from build123d import *

# Parameters (mm, degrees)
PAD_DEPTH       = 129
FILLET_R        = 3
FILLET001_R     = 2
POCKET_DEPTH    = 29.348127
SKETCH002_W     = 23
SKETCH002_H     = 7
POCKET001_DEPTH = 49


with BuildPart() as obj1:
    # Sketch → Pad (new body)
    with BuildSketch(Plane.XZ):
        with BuildLine():
            Line((0, 0), (0, 37))
            Line((0, 37), (3, 44))
            Line((3, 44), (3, 4))
            Line((3, 4), (26, 4))
            Line((26, 4), (21, 34))
            ThreePointArc((23.448856, 44), (21.197055, 39.251589), (21, 34))
            ThreePointArc((25.84203, 42.190943), (25.551614, 44.294231), (23.448856, 44))
            ThreePointArc((25.84203, 42.190943), (24.041555, 38.293355), (24.041381, 34))
            Line((24.041381, 34), (29.708048, 0))
            Line((29.708048, 0), (0, 0))
        make_face()
    extrude(amount=PAD_DEPTH)

    # Fillet
    fillet_edges = [obj1.edges().sort_by_distance(p)[0] for p in [
        (26, -64.5, 4),
        (3, -64.5, 4),
    ]]
    fillet(fillet_edges, radius=FILLET_R)

    # Fillet001
    fillet001_edges = [obj1.edges().sort_by_distance(p)[0] for p in [
        (0, -64.5, 0),
        (29.708048, -64.5, 0),
    ]]
    fillet(fillet001_edges, radius=FILLET001_R)

    # Sketch001 (on Face2 of Fillet001) → Pocket (cut, through all)
    with BuildSketch(Plane(origin=(0, 0, 0), x_dir=(0, 0, -1), z_dir=(-1, 0, 0))):
        Polygon((0, 49), (-45, 4), (-45, 0), (0, 0), align=None)
    extrude(amount=-POCKET_DEPTH, mode=Mode.SUBTRACT)

    # Sketch002 → Pocket001 (cut)
    with BuildSketch(Plane.XZ):
        with Locations((14.5, 3.5)):
            Rectangle(SKETCH002_W, SKETCH002_H)
    extrude(amount=POCKET001_DEPTH, mode=Mode.SUBTRACT)


with BuildPart() as part_mirroring:
    # Part__Mirroring: instance of obj1
    add(obj1.part.mirror(Plane(origin=(0, -129, 2), x_dir=(1, 0, 0), z_dir=(0, 1, 0))))


with BuildPart() as part_mirroring_1:
    # Part__Mirroring placement: moved
    add(part_mirroring.part.moved(Location((0, -35, 0))))


solid = part_mirroring_1.part
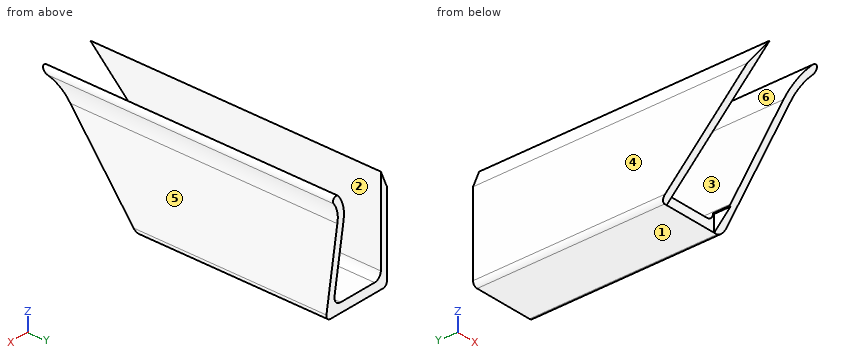
Geometry: final body of the model. Coordinates: model frame, mm. Face numbers are marked on the shaded views. A direction names the side the tool comes from. Coordinates: 2 decimals unless noted, no trailing zeros. Write each loop counter-clockwise with the first axis right and the second up, starting at its lowest first coordinate (ties: lowest second). Pieces come first, ordered by that corner, then holes. Notation, with made-up numbers: (53.5, 55.25) - (72.5, 55.25) arc R25 cw to (72.5, 90.25) - close; hole circle Ø8 at (-39.5, -14). An arc over 180 degrees is marked (long way). Return JSON: item names as keys, results as strings.
Item 1: Section query C-C (y = -214.5). Output: boundary loops of the cut face in (x, z).
Completed:
{"outline": "(0, 2) arc R2 ccw to (2, 0) - (27.35, 0) arc R2 ccw to (29.32, 2.33) - (24.04, 34) arc R10 cw to (25.84, 42.19) arc R1.5 ccw to (23.45, 44) arc R13.06 ccw to (21, 34) - (25.42, 7.49) arc R3 cw to (22.46, 4) - (6, 4) arc R3 cw to (3, 7) - (3, 44) - (0, 37) - close"}
Item 2: Pin query (flat end, axial travel): pin 1 Ø22 at (y, z) = (-227.5, 22) entering from +X; pin 2 Ø3 at (y, z) = (-189.5, 11) entering from +X; pin 3 Ø7.5 at (x, z) = (19.5, 5) entering from -Y; pin 4 Ø12 at (y, z) = (-225.5, 7.5) entering from +X. Return the tip coordinate at first contact, or that it passes through.
Completed:
{"pin 1": "stops at x = 27.87", "pin 2": "stops at x = 28.12", "pin 3": "stops at y = -244", "pin 4": "stops at x = 29.35"}
Item 3: Pull-direction query (Z, two-part tool) for the marked faces 1, 2 and 3; classes: +Z half, -Z half, draft (parallel to the pull), parting line (faces both ways), or undercut.
Completed:
{"face 1": "-Z half", "face 2": "draft", "face 3": "undercut"}
Item 4: Reachability of the marked faces 4, 5 and 6 from +Z, -Z, +X, -X, +Y, -Y: full face, straight path, thin tool, end or side. Return the list, or none.
Completed:
{"face 4": "+Z, -Z, -X, +Y, -Y", "face 5": "+X, +Y, -Y", "face 6": "+Y, -Y"}
Item 5: Line query: L1, parallel to X at y = -191.5, z = 34; L2, parallel to X at y = -216.5, z = 21; L3, parallel to Z at x = 17.75, y = -213. Output: solid intervals per line, ascending.
Completed:
{"L1": "x = 0 to 3, 21 to 24.04", "L2": "x = 0 to 3, 23.17 to 26.21", "L3": "z = 0 to 4"}
Item 6: Section query A-A (z = 24.5). Output: boundary loops of the cut face in (x, y), and give its area (3 significant figures).
Completed:
{"outline": "(0, -268.5) - (3, -268.5) - (3, -164) - (0, -164) - close; (22.58, -268.5) - (25.62, -268.5) - (25.62, -164) - (22.58, -164) - close", "area": "631 mm2"}
Item 7: Section query B-B (y = -253.5). Output: boundary loops of the cut face in (x, z), and give its area (3 significant figures).
Completed:
{"outline": "(0, 9.5) - (3, 9.5) - (3, 44) - (0, 37) - close; (21, 34) - (25.08, 9.5) - (28.12, 9.5) - (24.04, 34) arc R10 cw to (25.84, 42.19) arc R1.5 ccw to (23.45, 44) arc R13.06 ccw to start", "area": "200 mm2"}
Item 8: Section query D-D (z = 38.5). Output: boundary loops of the cut face in (x, y).
Completed:
{"outline": "(0.64, -282.5) - (3, -282.5) - (3, -164) - (0.64, -164) - close; (21.04, -282.5) - (24.09, -282.5) - (24.09, -164) - (21.04, -164) - close"}
